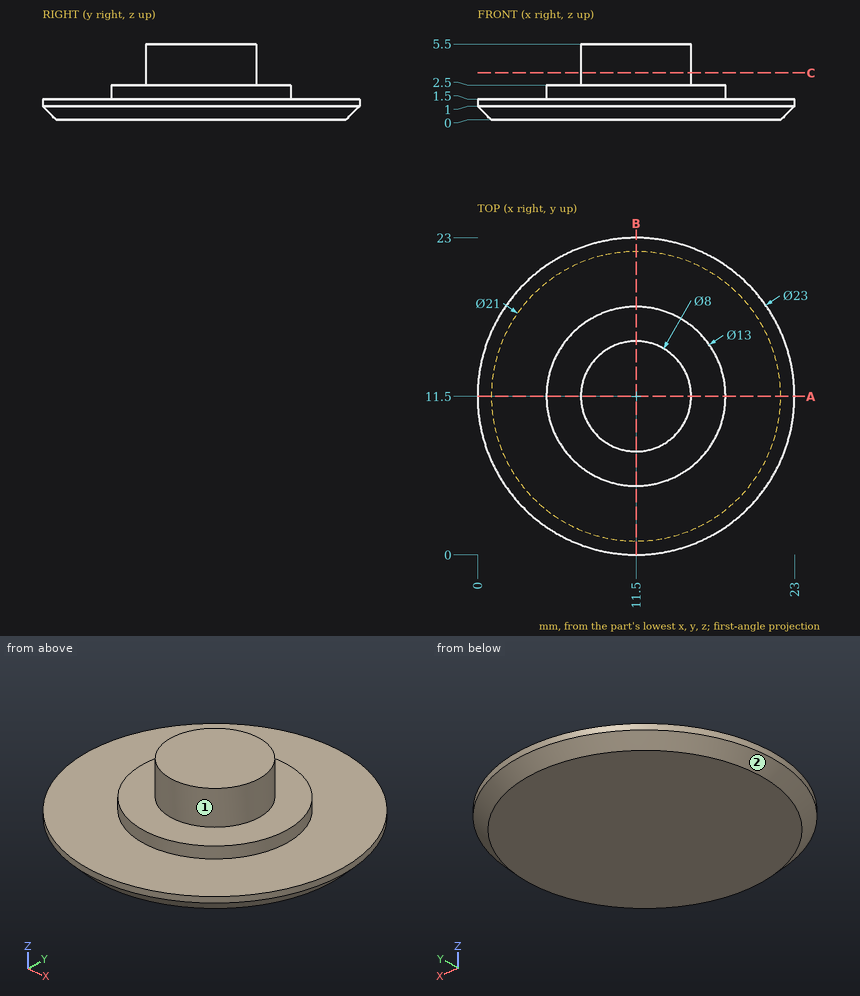
For this review, use the dimensioned drawing (mm, ordinates from the lowest corner) and the shaded views. A direction names the side the tool comes from. Give positions to 0.01 mm unless a question says otherwise; leave off trailing zeros. Order: outer loops, then holes, each group sorted by start corner. A loop starts at its lowest first (then second) coordinate and runs counter-clockwise, first axis right, second up. Notation, with made-up numbers: (66, 11.5) - (88, 11.5) arc R16 cw to (88, 42.5) - close; hole circle Ø1 at (24.25, 19.5). An arc over 180 degrees is marked (long way). Use a Markdown table: item, result. Add a question column.
(1) Add section C-C on z = 3.4. Give the boundary of the cut face in (x, y), then the cut area to 3 significant figures.
(2) Clearance check with flat-ended pins moving along their axes: P1, Ø1.5, axis at x = 12.5, y = 16.5, coming from the -Z side; P2, Ø1, axis at y = 3.5, z = 1, coming from the +X side; P3, Ø4, axis at x = 19.5, y = 9, coming from the +Z side; P4, Ø1, axis at y = 19, z = 1, coming from the -X side. State where each tip first meets the part, or that it passes through.
(3) Wall thickness on probe 1 along Z at (x, y) = (6.5, 19.75); probe 2 along Z at (x, y) = (9.25, 17.25); probe 3 along Y at (x, z) = (6.5, 0.35): over which ranges is each line inside the solid? List them lowest first. Write a range as [from, to].
(4) Add section A-A on y = 11.5. Give the boundary of the cut face in (x, z), then the cut area to 3 significant figures.
(5) Machinability: for the marked faces 1 and 2, which of the approach directions +Z, -Z, +X, -X, +Y, -Y give a long, thin tool a straight path to every point of the face, cutting with its end or side? Answer none if there is none.
Report:
| question | item | result |
|---|---|---|
| 1 | outline | circle Ø8 at (11.5, 11.5) |
| 1 | area | 50.3 mm² |
| 2 | P1 | stops at z = 0 |
| 2 | P2 | stops at x = 20.22 |
| 2 | P3 | stops at z = 2.5 |
| 2 | P4 | stops at x = 2.38 |
| 3 | probe 1 | z = [0, 1.5] |
| 3 | probe 2 | z = [0, 2.5] |
| 3 | probe 3 | y = [1.87, 21.13] |
| 4 | outline | (0, 1) - (1, 0) - (22, 0) - (23, 1) - (23, 1.5) - (18, 1.5) - (18, 2.5) - (15.5, 2.5) - (15.5, 5.5) - (7.5, 5.5) - (7.5, 2.5) - (5, 2.5) - (5, 1.5) - (0, 1.5) - close |
| 4 | area | 70.5 mm² |
| 5 | face 1 | +Z |
| 5 | face 2 | -Z |
